Geometry check sheet. Reference: the model listing, model coordinates, mm. A direction names the side the tool comes from. Give positions to 0.01 mm unless a question says otherwise; leave off trailing zeros. Order: outer loops, then holes, each group sorted by start corner. A loop starts at its lowest first (then second) coordinate and runs counter-clockwise, first axis right, second up. Notation, with made-up numbers: M 16,34.25 L 29,34.25 A21 ccw 29,46.25 Z; hole C -39,-39 d8. An arc over 180 degrees is marked long. Put each result on its own line as item: value. Start each with the question number.
Q1. Section check D-D on y = 5.25. Record the cut outline in (x, z).
Q2. Mould release check, pull along X, two halves, no side actions. Record for faces 1 (the cylindrical face through (21.3, 10.5, 13.6)), 2 (the cylindrical face through (-28.57, 6.08, 26)), 3 (the cylindrical face through (-7.412, 10.479, -10.002)), 4 (the cylindrical face through (28.5, 10.52, 26.07)): +X half, -X half, draft (parallel to the pull), parting line (faces both ways), or undercut.
Q3. Section check C-C on z = 12. Record the cut outline in (x, y), then the cut area to 3 significant figures.
Q4. Section check A-A on x = -7.5. Record the cut outline in (y, z), then the cut area to 3 significant figures.
Q5. Access from +Z, -Z, +X, -X, +Y, -Y to the whole of each face (thin tool, end or side, straight path). Record for faces 5 (the flat face through (-15, 4, 0)), 6 (the cylindrical face through (-28.57, 6.08, -26)).
Q6. Material ranges on L1, parallel to X at y = 11.45, z = 12; L2, parallel to X at y = 6.25, z = -20; L3, parallel to X at y = 5.5, z = 9, recorded low to high.
Q7. Go/stop test with flat-tipped pins: pin 1 (22.5 mm diameter, centred on x = 13.5, z = -8.5, fed in from -Y); pin 2 (7 mm diameter, centred on y = 4.5, z = 0.5, fed in from +X). Record where each tip stops, or that it passes through.
Q8. Section check B-B on z = 20. Record the cut outline in (x, y).
```python
from build123d import *

# Parameters (mm, degrees)
SKETCH1_W                 = 60
SKETCH1_H                 = 55
BOSS_EXTRUDE1_DEPTH       = 12
SKETCH2_W                 = 45
SKETCH2_H                 = 55
CUT_EXTRUDE2_DEPTH        = 9
M5_TAPPED_HOLE1_D         = 4.2
M5_TAPPED_HOLE1_DEPTH     = 12.4
M5_TAPPED_HOLE1_TIP       = 1.2618073
FILLET1_R                 = 5
F_4_0MM_DOWEL_HOLE2_D     = 4
F_4_0MM_DOWEL_HOLE2_DEPTH = 12.4
F_4_0MM_DOWEL_HOLE2_TIP   = 1.201721238


with BuildPart() as part:
    # Sketch1 → Boss-Extrude1 (new body)
    with BuildSketch(Plane(origin=(0, 0, 0), x_dir=(1, 0, 0), z_dir=(0, 1, 0))):
        Rectangle(SKETCH1_W, SKETCH1_H)
    extrude(amount=BOSS_EXTRUDE1_DEPTH)

    # Sketch2 → Cut-Extrude2 (cut)
    with BuildSketch(Plane.XZ):
        with Locations((7.5, 0)):
            Rectangle(SKETCH2_W, SKETCH2_H)
    extrude(amount=-CUT_EXTRUDE2_DEPTH, mode=Mode.SUBTRACT)

    # M5 Tapped Hole1
    with Locations(Plane(origin=(-25, 12, -20), x_dir=(0, 0, 1), z_dir=(0, 1, 0))):
        with Locations((0, 0), (40, 0)):
            Hole(M5_TAPPED_HOLE1_D / 2, depth=M5_TAPPED_HOLE1_DEPTH)
            with Locations((0, 0, -(M5_TAPPED_HOLE1_DEPTH + M5_TAPPED_HOLE1_TIP / 2))):  # 118° drill point
                Cone(0, M5_TAPPED_HOLE1_D / 2, M5_TAPPED_HOLE1_TIP, mode=Mode.SUBTRACT)

    # Fillet1
    fillet1_edges = [part.edges().sort_by_distance(p)[0] for p in [
        (30, 10.5, 27.5),
        (-30, 6, 27.5),
        (-30, 6, -27.5),
        (30, 10.5, -27.5),
    ]]
    fillet(fillet1_edges, radius=FILLET1_R)

    # Ø4.0mm Dowel Hole2
    with Locations(Plane(origin=(-7.5, 12, -12), x_dir=(0, 0, 1), z_dir=(0, 1, 0))):
        with Locations((0, 0), (24, 0), (24, 30), (0, 30)):
            Hole(F_4_0MM_DOWEL_HOLE2_D / 2, depth=F_4_0MM_DOWEL_HOLE2_DEPTH)
            with Locations((0, 0, -(F_4_0MM_DOWEL_HOLE2_DEPTH + F_4_0MM_DOWEL_HOLE2_TIP / 2))):  # 118° drill point
                Cone(0, F_4_0MM_DOWEL_HOLE2_D / 2, F_4_0MM_DOWEL_HOLE2_TIP, mode=Mode.SUBTRACT)


solid = part.part
```
Results found:
1. outline: M -30,-22.5 A5 ccw -25,-27.5 L -15,-27.5 L -15,27.5 L -25,27.5 A5 ccw -30,22.5 Z; hole C -25,-20 d4.2; hole C -25,20 d4.2
2. face 1: undercut
2. face 2: -X half
2. face 3: undercut
2. face 4: +X half
3. outline: M -30,0 L -15,0 L -15,9 L -9.5,9 L -9.5,12 L -30,12 Z; M -5.5,9 L 20.5,9 L 20.5,12 L -5.5,12 Z; M 24.5,9 L 30,9 L 30,12 L 24.5,12 Z
3. area: 291 mm^2
4. outline: M 9,-27.5 L 12,-27.5 L 12,-14 L 9,-14 Z; M 9,-10 L 12,-10 L 12,10 L 9,10 Z; M 9,14 L 12,14 L 12,27.5 L 9,27.5 Z
4. area: 141 mm^2
5. face 5: +Z, -Z, +X, -Y
5. face 6: -Z, -X, +Y, -Y
6. L1: x = -30 to -9.5, -5.5 to 20.5, 24.5 to 30
6. L2: x = -30 to -27.1, -22.9 to -15
6. L3: x = -30 to -15
7. pin 1: stops at y = 9
7. pin 2: stops at x = -15
8. outline: M -30,0 L -27.1,0 L -27.1,12 L -30,12 Z; M -22.9,0 L -15,0 L -15,9 L 30,9 L 30,12 L -22.9,12 Z
